Work out the finished part from the listing and answer in its coordinate system (mm). Face numbers are marked on the shaded views. A direction names the side the tool comes from. Coordinates: 2 decimals unless noted, no trailing zeros. Order: outer loops, then holes, each group sorted by start corner. A loop starts at its lowest first (then second) coordinate and runs counter-clockwise, first axis right, second up.
1. The part is cut by section A-A, the plane y = 0. Give the vertices of the cut face in (x, z), then the cut area to 3 significant figures.
2. Find the intervals of material crossed by probe 1 along Y at (x, z) = (-1, -23); probe 2 along Z at (x, y) = (-23.5, -0.5); probe 3 along Z at (x, y) = (31.5, -26.5), in increasing order.
3. A tool of negligible diameter and unlimited length cuts with its end or side. For the marked faces 1, 2 and 3, from which of +Z, -Z, +X, -X, +Y, -Y can it reach the whole face along a straight path? Write none if from no direction.
4. Flat-ended cylindrical pins translate along their axes: pin 1 Ø5 at (x, z) = (30, -17.5) entering from -Y; pin 2 Ø3 at (y, z) = (-6, -5.5) entering from -X; pin 3 Ø5 at (x, z) = (-10.5, -63.5) entering from -Y. Find the tip coordinate at first contact, or state that the pin passes through.
5. The part is cut by section B-B, the plane x = -28. Give the vertices of the cut face in (y, z).
6. The part is cut by section C-C, the plane z = -83.5. Give the vertices of the cut face in (x, y), then the cut area to 3 significant figures.
```python
from build123d import *

# Parameters (mm, degrees)
F0_R     = 21.212029
F1_DEPTH = 17.26026
F2_R     = 44.593298
F3_DEPTH = 71.53698
F4_R     = 31.424111
F5_DEPTH = 91.14636


with BuildPart() as f1:
    # F0 (on Top) → F1 (new body)
    with BuildSketch(Plane.XY):
        Circle(F0_R)
    extrude(amount=F1_DEPTH)

    # F2 (on Top) → F3 (join)
    with BuildSketch(Plane.XY):
        Circle(F2_R)
    extrude(amount=-F3_DEPTH)

    # F4 (on Top) → F5 (join)
    with BuildSketch(Plane.XY):
        Circle(F4_R)
    extrude(amount=-F5_DEPTH)


solid = f1.part
```
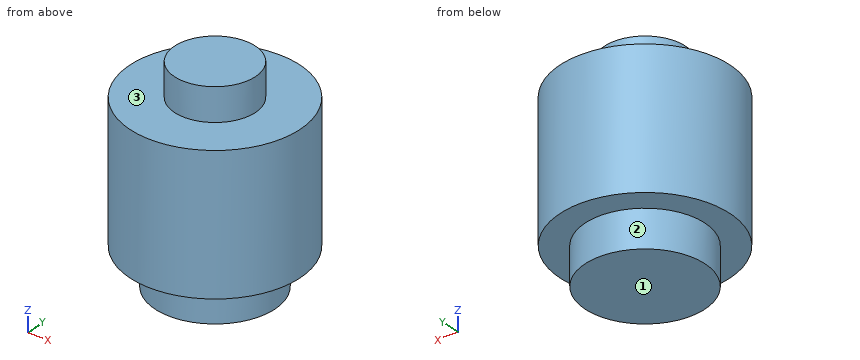
Geometry says:
1. outline: (-44.59, -71.54) - (-31.42, -71.54) - (-31.42, -91.15) - (31.42, -91.15) - (31.42, -71.54) - (44.59, -71.54) - (44.59, 0) - (21.21, 0) - (21.21, 17.26) - (-21.21, 17.26) - (-21.21, 0) - (-44.59, 0) - close
1. area: 8,340 mm2
2. probe 1: y = -44.58 to 44.58
2. probe 2: z = -91.15 to 0
2. probe 3: z = -71.54 to 0
3. face 1: -Z, +X, -X, +Y, -Y
3. face 2: -Z
3. face 3: +Z
4. pin 1: stops at y = -35.1
4. pin 2: stops at x = -44.37
4. pin 3: stops at y = -43.87
5. outline: (-34.71, -71.54) - (-14.26, -71.54) - (-14.26, -91.15) - (14.26, -91.15) - (14.26, -71.54) - (34.71, -71.54) - (34.71, 0) - (-34.71, 0) - close
6. outline: circle Ø62.85 at (0, 0)
6. area: 3,100 mm2
